```python
from build123d import *

# Parameters (mm, degrees)
CROQUIS1_R              = 17
SALIENTE_EXTRUIR1_DEPTH = 30
CORTAR_EXTRUIR5_DEPTH   = 66.901748436


with BuildPart() as part:
    # Croquis1 → Saliente-Extruir1 (new body)
    with BuildSketch(Plane.XY):
        with BuildLine():
            Line((-34.751366554, 8.708761257), (-8.067498219, 19.65904302))
            ThreePointArc((-8.067498219, 19.65904302), (9.932956283, 18.785602984), (20.78928746, 4.400912053))
            ThreePointArc((20.78928746, 4.400912053), (21.824692428, 2.04462752), (23.714959375, 0.297907417))
            Line((23.714959375, 0.297907417), (43.380202362, -11.504419481))
            Line((43.380202362, -11.504419481), (37.980772654, -20.60816348))
            Line((37.980772654, -20.60816348), (29.126956343, -16.414809963))
            ThreePointArc((29.126956343, -16.414809963), (20.290915471, -14.763720087), (11.788304563, -17.680451791))
            ThreePointArc((11.788304563, -17.680451791), (-0.239292664, -21.24865264), (-12.18348282, -17.410492422))
            ThreePointArc((-12.18348282, -17.410492422), (-18.624029112, -14.886802036), (-25.506269787, -15.582799871))
            ThreePointArc((-25.506269787, -15.582799871), (-41.965765273, -7.942029126), (-34.751366554, 8.708761257))
        make_face()
        Circle(CROQUIS1_R, mode=Mode.SUBTRACT)
    extrude(amount=SALIENTE_EXTRUIR1_DEPTH)

    # Croquis7 → Cortar-Extruir5 (cut, through all)
    with BuildSketch(Plane(origin=(6.411424524, 10.682827398, 0), x_dir=(0.857431728196329, -0.5145977375409424, 0), z_dir=(0.5145977375409424, 0.857431728196329, 0))):
        with BuildLine():
            Line((20.180656118, 0), (20.180656118, 9.238458875))
            Line((20.180656118, 9.238458875), (56.582580984, 4.619229438))
            Line((56.582580984, 4.619229438), (52.496685568, -37.874416839))
            Line((52.496685568, -37.874416839), (21.89416276, -35.456233837))
            Line((21.89416276, -35.456233837), (20.180656118, -30))
            Line((20.180656118, -30), (36.352428356, -24.467854313))
            ThreePointArc((36.352428356, -24.467854313), (43.115709537, -15.009568923), (36.358878018, -5.546674933))
            Line((36.358878018, -5.546674933), (20.180656118, 0))
        make_face()
    extrude(amount=-CORTAR_EXTRUIR5_DEPTH, mode=Mode.SUBTRACT)


solid = part.part
```
Geometry: final body of the model. Coordinates: model frame, mm. A direction names the side the tool comes from. Round coordinates to 2 decimals unless told otherwise and drop trailing zeros. Loops run counter-clockwise (first coordinate to the right, second up) from the corner with the lowest first, then second, coordinate; pieces in that order, holes last. Notation, with made-up numbers: (71, 66) -> (130, 66) arc R26 cw to (130, 105) -> close; hole circle Ø4 at (44.5, 37). An arc over 180 degrees is marked (long way). Write each question's results on one line, items separated by ' | '.
Item 1: Pin query (flat end, axial travel): pin 1 Ø2 at (y, z) = (13.5, 24.5) entering from -X; pin 2 Ø10 at (y, z) = (-1.5, 3) entering from +X; pin 3 Ø3 at (x, z) = (2.5, 22) entering from +Y; pin 4 Ø5 at (x, y) = (1.5, 16.5) entering from +Z. Return the tip coordinate at first contact, or that it passes through.
Answers below:
pin 1: stops at x = -25.51 | pin 2: stops at x = 34.71 | pin 3: stops at y = 21.23 | pin 4: stops at z = 30
Item 2: Pull-direction query (X, two-part tool) for faces 1 (the face through (31.225, -4.209, 14.79)), 2 (the face through (9.139, 14.334, 14.79)), 3 (the face through (-16.5, 5, 0)); classes: pulls with the +X half, pulls with the -X half, needs draft (parallel to the pull), parting line crosses it, or undercut.
Answers below:
face 1: pulls with the +X half | face 2: undercut | face 3: needs draft
Item 3: Set-up query: faces 4 (the face through (32.612, -18.066, 14.859)), 5 (the face through (21.804, 2.074, 14.79)). Return all of +Z, -Z, +X, -X, +Y, -Y with unobstructed straight access to the full face (end or side cutting, diameter ignored); none if empty.
Answers below:
face 4: +Z, -Z, -Y | face 5: +Z, -Z, +X, +Y
Item 4: Cut plane C-C on y = 2. Return the cut outline in (x, z).
Answers below:
outline: (-41.68, 0) -> (-16.88, 0) -> (-16.88, 30) -> (-41.68, 30) -> close; (16.88, 0) -> (21.86, 0) -> (21.86, 30) -> (16.88, 30) -> close
Item 5: Cut plane B-B on z = 27.5. Return the cut outline in (x, y).
Answers below:
outline: (-34.75, 8.71) arc R13 ccw to (-25.51, -15.58) arc R14.72 cw to (-12.18, -17.41) arc R21.25 ccw to (11.79, -17.68) arc R17.64 cw to (23.18, -14.79) -> (29.98, -3.46) -> (23.71, 0.3) arc R6.31 cw to (20.79, 4.4) arc R21.25 ccw to (-8.07, 19.66) -> close; hole circle Ø34 at (0, 0)
Item 6: Cut plane A-A on x = 0. Return the cut outline in (y, z).
Answers below:
outline: (-21.25, 0) -> (-17, 0) -> (-17, 30) -> (-21.25, 30) -> close; (17, 0) -> (21.25, 0) -> (21.25, 30) -> (17, 30) -> close
Item 7: Line query: probe 1 along Y at (x, z) = (0, 15.25); probe 2 along X at (y, z) = (-11, 14.5); probe 3 along X at (y, z) = (15, 3). Output: solid intervals per line, ascending. Write a range as [from, to].
Answers below:
probe 1: y = [-21.25, -17], [17, 21.25] | probe 2: x = [-40.3, -12.96], [12.96, 42.54] | probe 3: x = [-19.42, -8], [8, 15.05]
Item 8: Cut plane D-D on z = 19.5. Return the cut outline in (x, y).
Answers below:
outline: (-34.75, 8.71) arc R13 ccw to (-25.51, -15.58) arc R14.72 cw to (-12.18, -17.41) arc R21.25 ccw to (11.79, -17.68) arc R17.64 cw to (29.13, -16.41) -> (36.96, -20.13) -> (42.47, -10.96) -> (23.71, 0.3) arc R6.31 cw to (20.79, 4.4) arc R21.25 ccw to (-8.07, 19.66) -> close; hole circle Ø34 at (0, 0)
